```python
from build123d import *

# Parameters (mm, degrees)
F0_W        = 50
F0_H        = 6
F0_H_2      = 2
F1_DEPTH    = 2
F2_DEPTH    = 5
F3_T1_DEPTH = 70


# Not quite as in the source:
# - a fillet or chamfer that OpenCascade refuses, or shapes differently, is made with other operations: its cross-section is extruded or revolved along the edge and cut away or added
# - a feature names something its author has since deleted; it is built from what else it names


with BuildPart() as f1:
    # F0 (on Top) → F1 (new body)
    with BuildSketch(Plane.XY):
        Rectangle(F0_W, F0_H)
        with Locations((0, 4)):
            Rectangle(F0_W, F0_H_2)
        with Locations((0, -4)):
            Rectangle(F0_W, F0_H_2)
    extrude(amount=F1_DEPTH)

    # F0 (on Top) → F2 (join)
    with BuildSketch(Plane.XY):
        with Locations((0, 4)):
            Rectangle(F0_W, F0_H_2)
        with Locations((0, -4)):
            Rectangle(F0_W, F0_H_2)
    extrude(amount=F2_DEPTH)

    # F3: fillet of radius 5 on 2 edges, made by hand

    # F3_s2 → F3_t1 (cut)
    with BuildSketch(Plane.YZ.offset(-35)):
        with BuildLine():
            ThreePointArc((-5, 1), (-4.472135955, 3.2360679775), (-3, 5))
            Line((-3, 5), (-5, 5))
            Line((-5, 5), (-5, 1))
        make_face()
        with BuildLine():
            ThreePointArc((5, 1), (4.472135955, 3.2360679775), (3, 5))
            Line((3, 5), (5, 5))
            Line((5, 5), (5, 1))
        make_face()
    extrude(amount=F3_T1_DEPTH, mode=Mode.SUBTRACT)


solid = f1.part
```
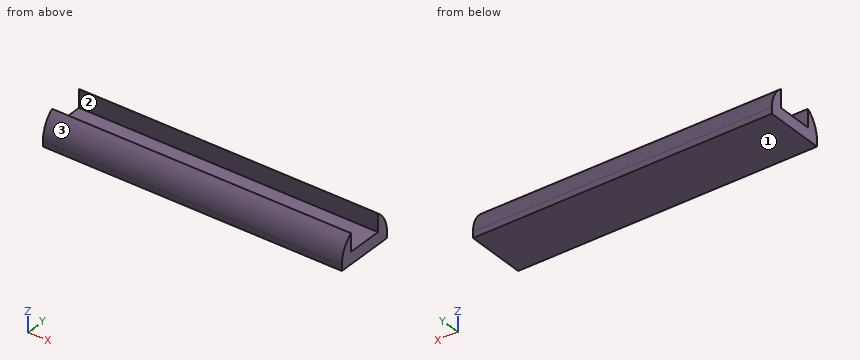
Part model, mm, in its own coordinate system. Face numbers are marked on the shaded views. Round coordinates to 2 decimals unless told otherwise and drop trailing zeros. Order: outer loops, then holes, each group sorted by start corner. A loop starts at its lowest first (then second) coordinate and runs counter-clockwise, first axis right, second up. Notation, with made-up numbers: M 84,71.25 L 104,71.25 A27 cw 104,96.25 Z; hole C 67.25,-18.75 d3. An arc over 180 degrees is marked long. Answer in a Markdown table with one row per item. Add a question column.
Q1. Cut at B-B on x = -16. Give the cut face in (y, z), and give its area (3 significant figures).
Q2. Mould opens along Y. For the marked faces 1, 2 and 3 say: +Y half, -Y half, draft (parallel to the pull), parting line (faces both ways), or undercut.
Q3. Pin check, flat tips, straight feed: pin 1 (1.5 mm diameter, centred on x = 10.5, y = 0, fed in from +Z); pin 2 (1.5 mm diameter, centred on x = -8, z = 3.5, fed in from -Y); pin 3 (1.5 mm diameter, centred on x = -10, z = 3, fed in from +Y). Stop position of each tip, or through.
Q4. Cut at C-C on y = 4. Give the cut face in (x, z), and give its area (3 significant figures).
Q5. Cut at A-A on z = 3.25. Give the cut face in (x, y), and give its area (3 significant figures).
Q6. Wall check: L1, parallel to Y at x = 1.5, z = 3.9; L2, parallel to Y at x = 20, z = 2.2; L3, parallel to Z at x = -8.5, y = 2.75. Give the ranges that are in metal, low to high. Write a range as from..to.
Established:
| question | item | result |
|---|---|---|
| 1 | outline | M -5,0 L 5,0 L 5,1 A5 ccw 3,5 L 3,2 L -3,2 L -3,5 A5 ccw -5,1 Z |
| 1 | area | 27.2 mm2 |
| 2 | face 1 | draft |
| 2 | face 2 | undercut |
| 2 | face 3 | -Y half |
| 3 | pin 1 | stops at z = 2 |
| 3 | pin 2 | stops at y = -4.68 |
| 3 | pin 3 | stops at y = 4.84 |
| 4 | outline | M -25,0 L 25,0 L 25,4 L -25,4 Z |
| 4 | area | 200 mm2 |
| 5 | outline | M -25,-4.47 L 25,-4.47 L 25,-3 L -25,-3 Z; M -25,3 L 25,3 L 25,4.47 L -25,4.47 Z |
| 5 | area | 147 mm2 |
| 6 | L1 | y = -4.07..-3, 3..4.07 |
| 6 | L2 | y = -4.85..-3, 3..4.85 |
| 6 | L3 | z = 0..2 |
